Source: three-view drawing plus pictorial views. Frame: mm from the lowest corner of the part. A direction names the side the tool comes from. Give positions to 0.01 mm unless a question says otherwise; leave off trailing zeros. Order: outer loops, then holes, each group sorted by start corner. A loop starts at its lowest first (then second) coordinate and runs counter-clockwise, first axis right, second up.
1) Material intervals for line 1 (X direction, y = 24, z = 3.7); line 2 (Y direction, x = 17.5, z = 4.75); line 3 (X direction, y = 13, z = 4.6), sorted ascending.
2) Section B-B, the plane y = 24. Return loops of the section in (x, z).
3) Section C-C, the plane x = 5. Return loops of the section in (y, z).
4) First-contact query: P1, Ø3, axis at y = 11.5, z = 3, coming from the -X side; P2, Ø9, axis at x = 14.5, y = 25, coming from the -Z side; P3, Ø1, axis at x = 9, z = 4, coming from the -Y side. Flat tips, straight axial feed; report the tip coordinate or a pass-through.
5) Section A-A, the plane z = 4.65. Return loops of the section in (x, y).
6) Access query for the marked faces 4, 5 and 6. Directions: +Z, -Z, +X, -X, +Y, -Y. A direction counts if a zero-diameter tool reaches every point of the face in a straight line with its end or side. Return the directions, or none.
7) Draft query along Y for the marked faces 1, 2 and 3. Return one class per face: released by +Y, released by -Y, zero draft, split by the parting line, or undercut.
8) Section D-D, the plane y = 14. Return loops of the section in (x, z).
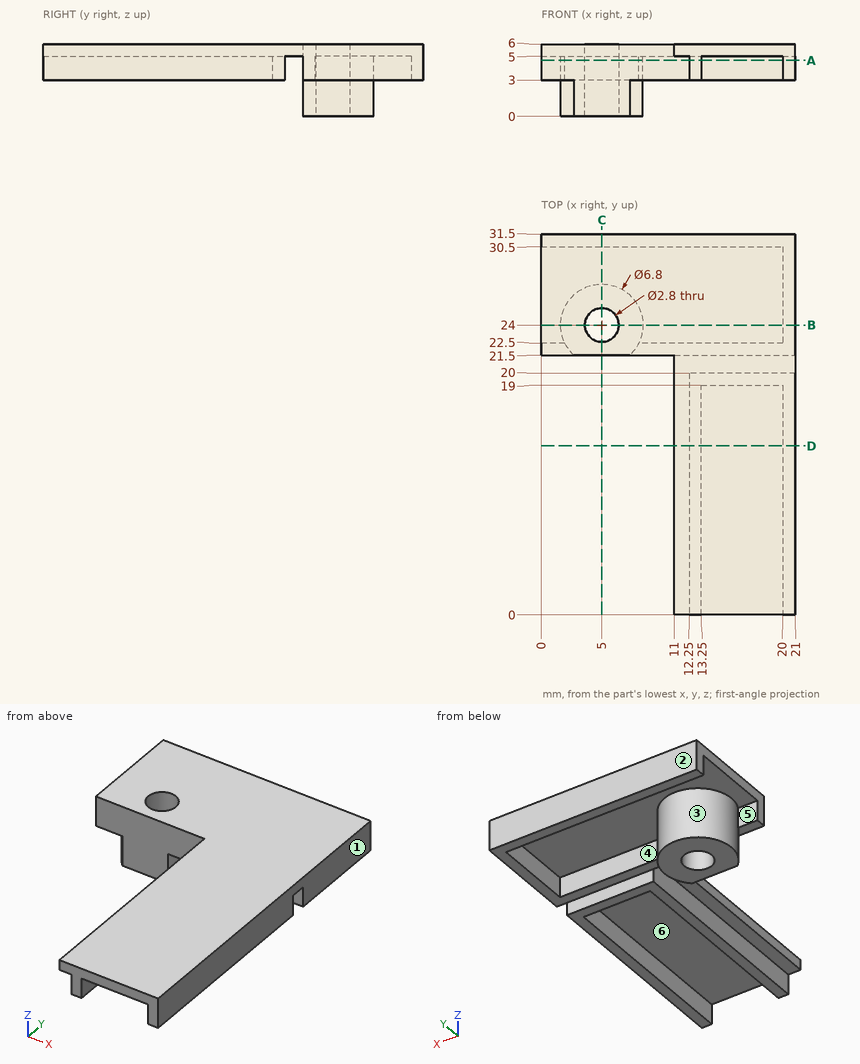
From the geometry:
1. line 1: x = 1.6 to 3.6, 6.4 to 8.4, 20 to 21
1. line 2: y = 19 to 20, 21.5 to 22.5, 30.5 to 31.5
1. line 3: x = 12.25 to 13.25, 20 to 21
2. outline: (0, 5) - (1.6, 5) - (1.6, 0) - (3.6, 0) - (3.6, 6) - (0, 6) - close; (6.4, 0) - (8.4, 0) - (8.4, 5) - (20, 5) - (20, 3) - (21, 3) - (21, 6) - (6.4, 6) - close
3. outline: (21.5, 0) - (22.6, 0) - (22.6, 6) - (21.5, 6) - close; (25.4, 0) - (27.4, 0) - (27.4, 5) - (30.5, 5) - (30.5, 3) - (31.5, 3) - (31.5, 6) - (25.4, 6) - close
4. P1: stops at x = 12.25
4. P2: stops at z = 3
4. P3: stops at y = 21.5
5. outline: (0, 21.5) - (21, 21.5) - (21, 31.5) - (0, 31.5) - (0, 30.5) - (20, 30.5) - (20, 22.5) - (8.05, 22.5) arc R3.4 ccw (long way) to (1.95, 22.5) - (0, 22.5) - close; (12.25, 0) - (13.25, 0) - (13.25, 19) - (20, 19) - (20, 0) - (21, 0) - (21, 20) - (12.25, 20) - close; hole circle Ø2.8 at (5, 24)
6. face 4: -Z
6. face 5: -Z, -X
6. face 6: -Z, -Y
7. face 1: zero draft
7. face 2: released by +Y
7. face 3: undercut
8. outline: (11, 5) - (12.25, 5) - (12.25, 3) - (13.25, 3) - (13.25, 5) - (20, 5) - (20, 3) - (21, 3) - (21, 6) - (11, 6) - close
